For this review, take the finished solid that the model builds, in its own axes (mm). A direction names the side the tool comes from. Round coordinates to 2 decimals unless told otherwise and drop trailing zeros. Order: outer loops, then holes, each group sorted by start corner. A loop starts at its lowest first (then second) coordinate and runs counter-clockwise, first axis right, second up.
from build123d import *

# Parameters (mm, degrees)
SKETCH1_W           = 41
SKETCH1_H           = 12
BOSS_EXTRUDE1_DEPTH = 4
SKETCH2_R           = 9.5
SKETCH2_R_2         = 2.6
BOSS_EXTRUDE2_DEPTH = 4
SKETCH3_R           = 5.05
BOSS_EXTRUDE3_DEPTH = 4
SKETCH4_R           = 5.05
BOSS_EXTRUDE4_DEPTH = 4
SKETCH5_W           = 10.1
SKETCH5_H           = 23.124939501
BOSS_EXTRUDE5_DEPTH = 4
SKETCH6_W           = 42
SKETCH6_H           = 12
SKETCH6_R           = 1.7
BOSS_EXTRUDE6_DEPTH = 2.5
SKETCH7_R           = 2.6
CUT_EXTRUDE1_DEPTH  = 4
SKETCH8_R           = 5.05
BOSS_EXTRUDE7_DEPTH = 2.7
SKETCH9_R           = 2.05
CUT_EXTRUDE2_DEPTH  = 6.7


with BuildPart() as part:
    # Sketch1 → Boss-Extrude1 (new body)
    with BuildSketch(Plane.XY.offset(358.5)):
        with Locations((298.5, 36)):
            Rectangle(SKETCH1_W, SKETCH1_H)
    extrude(amount=BOSS_EXTRUDE1_DEPTH)

    # Sketch2 → Boss-Extrude2 (add)
    with BuildSketch(Plane.XY.offset(358.5)):
        with Locations((300, 40)):
            Circle(SKETCH2_R)
        with Locations((300, 40)):
            Circle(SKETCH2_R_2, mode=Mode.SUBTRACT)
    extrude(amount=BOSS_EXTRUDE2_DEPTH)

    # Sketch4 → Boss-Extrude4 (add)
    with BuildSketch(Plane.XY.offset(358.5)):
        with Locations((280.050647312, 41.422437104)):
            Circle(SKETCH4_R)
    extrude(amount=BOSS_EXTRUDE4_DEPTH)



with BuildPart() as body_2:
    # Sketch3 → Boss-Extrude3 (new body)
    with BuildSketch(Plane.XY.offset(358.5)):
        with Locations((315.090923202, 53.124939501)):
            Circle(SKETCH3_R)
    extrude(amount=BOSS_EXTRUDE3_DEPTH)


with BuildPart() as part_1:
    add(part.part)

    add(body_2.part)  # Boss-Extrude5 merges body 2
    # Sketch5 → Boss-Extrude5 (add)
    with BuildSketch(Plane.XY.offset(358.5)):
        with Locations((315.090923202, 41.562469751)):
            Rectangle(SKETCH5_W, SKETCH5_H)
    extrude(amount=BOSS_EXTRUDE5_DEPTH)

    # Sketch6 → Boss-Extrude6 (add)
    with BuildSketch(Plane(origin=(0, 30, 0), x_dir=(1, 0, 0), z_dir=(0, 1, 0))):
        with Locations((300, -368.5)):
            Rectangle(SKETCH6_W, SKETCH6_H)
        with Locations(Location((285, -369.5, 0), (0, 0, 270))):
            Circle(SKETCH6_R, mode=Mode.SUBTRACT)
        with Locations(Location((315, -369.5, 0), (0, 0, 270))):
            Circle(SKETCH6_R, mode=Mode.SUBTRACT)
    extrude(amount=BOSS_EXTRUDE6_DEPTH)

    # Sketch7 → Cut-Extrude1 (cut)
    with BuildSketch(Plane.XY.offset(358.5)):
        with Locations((300, 40)):
            Circle(SKETCH7_R)
    extrude(amount=CUT_EXTRUDE1_DEPTH, mode=Mode.SUBTRACT)

    # Sketch8 → Boss-Extrude7 (add)
    with BuildSketch(Plane.XY.offset(362.5)):
        with Locations((315.090923202, 53.124939501)):
            Circle(SKETCH8_R)
        with Locations(Location((280.050647312, 41.422437104, 0), (0, 0, 246.041880591))):
            Circle(SKETCH8_R)
    extrude(amount=BOSS_EXTRUDE7_DEPTH)

    # Sketch9 → Cut-Extrude2 (cut)
    with BuildSketch(Plane.XY.offset(358.5)):
        with Locations(Location((315.090923202, 53.124939501, 0), (0, 0, 180))):
            Circle(SKETCH9_R)
        with Locations(Location((280.050647312, 41.422437104, 0), (0, 0, 180))):
            Circle(SKETCH9_R)
    extrude(amount=CUT_EXTRUDE2_DEPTH, mode=Mode.SUBTRACT)


solid = part_1.part
(1) Add section A-A on x = 300. Give the boundary of the cut face in (y, z), plus the area to 3 significant figures.
(2) Add section D-D on y = 40. Give the boundary of the cut face in (x, z), plus the area to 3 significant figures.
(3) Draft analysis for pull direction Y (two halves, no side actions). For faces 5 (the face through (314.43, 58.13, 362.55)), 6 (the face through (299, 30, 366)), 7 (the face through (300, 31, 374.5)), state which applies: pulls with the +Y half, pulls with the -Y half, needs draft (parallel to the pull), parting line crosses it, or undercut.
(4) Wall thickness on L1, parallel to X at y = 31.55, z = 369.5; L2, parallel to Z at x = 285, y = 31.35; L3, parallel to Y at x = 300, z = 360.45: over which ranges is each line inside the solid? List them lowest first.
(5) Tool access review of faces 1 (the face through (275.99, 44.425, 361.803)), 2 (the face through (317.3, 53.2, 365.2)), 3 (the face through (310.041, 47, 360)), 4 (the face through (279, 31, 369)): name each direction out of +Z, -Z, +X, -X, +Y, -Y from which nothing blocks a thin tool from reaching the whole face with its end or side.
(6) Add section C-C on x = 315. Give the boundary of the cut face in (y, z).
(7) Add section B-B on z = 370.25. Give the boundary of the cut face in (x, y), plus the area to 3 significant figures.
(8) Clearance check with flat-ended pins moving along their axes: P1, Ø4.5, axis at y = 34.5, z = 361.5, coming from the -X side; P2, Ø5, axis at x = 278.5, y = 41, coming from the +Z side; P3, Ø8, axis at y = 53.5, z = 362.5, coming from the +X side. State where each tip first meets the part, or that it passes through.
Here are the results:
1. outline: (30, 358.5) - (37.4, 358.5) - (37.4, 362.5) - (32.5, 362.5) - (32.5, 374.5) - (30, 374.5) - close; (42.6, 358.5) - (49.5, 358.5) - (49.5, 362.5) - (42.6, 362.5) - close
1. area: 87.2 mm2
2. outline: (275.21, 358.5) - (278.57, 358.5) - (278.57, 365.2) - (275.21, 365.2) - close; (281.53, 358.5) - (297.4, 358.5) - (297.4, 362.5) - (284.9, 362.5) - (284.9, 365.2) - (281.53, 365.2) - close; (302.6, 358.5) - (320.14, 358.5) - (320.14, 362.5) - (302.6, 362.5) - close
2. area: 165 mm2
3. face 5: undercut
3. face 6: pulls with the -Y half
3. face 7: needs draft
4. L1: x = 279 to 283.3, 286.7 to 313.3, 316.7 to 321
4. L2: z = 358.5 to 367.8, 371.2 to 374.5
4. L3: y = 30 to 37.4, 42.6 to 49.5
5. face 1: +Z
5. face 2: +Z, +X, -X, +Y
5. face 3: +Z, -Z, +Y
5. face 4: +Z, -X, -Y
6. outline: (30, 358.5) - (51.08, 358.5) - (51.08, 365.2) - (48.08, 365.2) - (48.08, 362.5) - (32.5, 362.5) - (32.5, 367.8) - (30, 367.8) - close; (30, 371.2) - (32.5, 371.2) - (32.5, 374.5) - (30, 374.5) - close; (55.17, 358.5) - (58.17, 358.5) - (58.17, 365.2) - (55.17, 365.2) - close
7. outline: (279, 30) - (283.47, 30) - (283.47, 32.5) - (279, 32.5) - close; (286.53, 30) - (313.47, 30) - (313.47, 32.5) - (286.53, 32.5) - close; (316.53, 30) - (321, 30) - (321, 32.5) - (316.53, 32.5) - close
7. area: 89.7 mm2
8. P1: stops at x = 278
8. P2: stops at z = 365.2
8. P3: stops at x = 320.14
